Answer from the drawing. Dimensions are ordinates in mm from the lowest x, y and z of the part. A direction names the side the tool comes from. Coordinates: 2 decimals unless noted, no trailing zeros. Write each loop counter-clockwise with the first axis right and the second up, starting at its lowest first coordinate (ties: lowest second). Pieces come first, ordered by that corner, then holes. Notation, with made-up numbers: (25, -16.75) -> (56, -16.75) arc R9 ccw to (56, -5.75) -> close; hole circle Ø10 at (1.5, 55). An arc over 180 degrees is marked (long way). One line per item, written item: value. Start each with the question number.
1. Find section A-A, the plane z = 3.5. Write down the section's boundary in (x, y), and give its area (3 significant figures).
2. Consider line 1 along X through (y, z) = (2.65, 32.5); line 2 along Z through (x, y) = (16.25, 3.75); line 3 along Z through (x, y) = (6.75, 2.75). Determine where each line is inside the solid, lowest interval first.
3. For the marked faces 1, 2 and 3, determine the directions among +Z, -Z, +X, -X, +Y, -Y from which every point of the face is accessible in a straight line to the end or side of a thin tool.
4. Find section B-B, the plane x = 16. State how many separate pieces and enclosed holes the cut face has, and give its area (3 significant figures).
5. Given P1, Ø0.9, axis at x = 8, y = 5, coming from the -Z side; P2, Ø3, axis at x = 12, z = 4, coming from the +Y side; P3, Ø1, axis at x = 8, z = 21.5, coming from the -Y side; P4, Ø3, axis at x = 4, z = 32.5, coming from the +Y side, each flat-ended and moving along its own axis, determine where each tip first touches the part or whether it passes through.
6. Find section C-C, the plane y = 3.5. Write down the section's boundary in (x, z).
7. Find section D-D, the plane x = 13.5. Write down the section's boundary in (y, z).
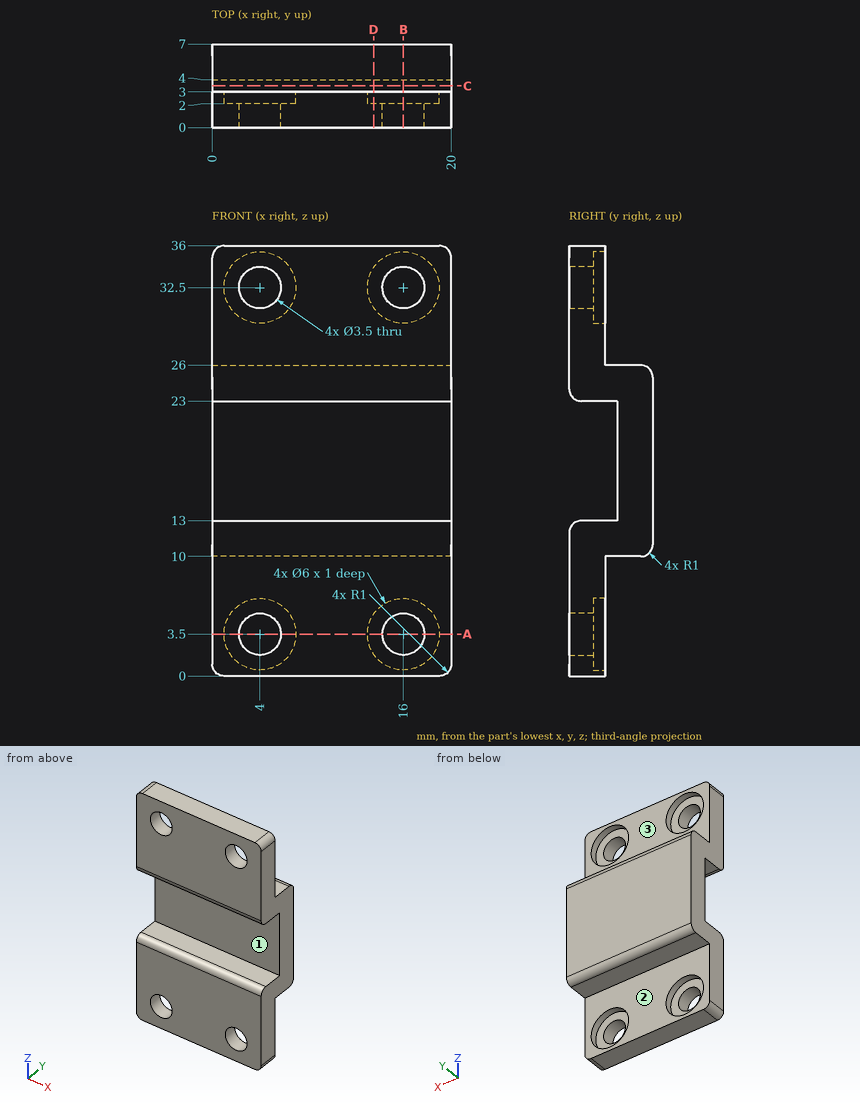
Answer block:
1. outline: (0, 0) -> (2.25, 0) -> (2.25, 2) -> (1, 2) -> (1, 3) -> (0, 3) -> close; (5.75, 0) -> (14.25, 0) -> (14.25, 2) -> (13, 2) -> (13, 3) -> (7, 3) -> (7, 2) -> (5.75, 2) -> close; (17.75, 0) -> (20, 0) -> (20, 3) -> (19, 3) -> (19, 2) -> (17.75, 2) -> close
1. area: 34.0 mm2
2. line 1: x = 0 to 1, 7 to 13, 19 to 20
2. line 2: z = 10 to 13, 23 to 26
2. line 3: z = 0 to 2.3, 4.7 to 13, 23 to 31.3, 33.7 to 36
3. face 1: +X, -X, -Y
3. face 2: -Z, +X, -X, +Y
3. face 3: +Z, +X, -X, +Y
4. separate pieces: 3
4. enclosed holes: 0
4. area: 105 mm2
5. P1: stops at z = 10
5. P2: stops at y = 3
5. P3: stops at y = 4
5. P4: passes through
6. outline: (0, 10) -> (20, 10) -> (20, 13) -> (0, 13) -> close; (0, 23) -> (20, 23) -> (20, 26) -> (0, 26) -> close
7. outline: (0, 0) -> (3, 0) -> (3, 1.84) -> (2, 1.84) -> (2, 5.16) -> (3, 5.16) -> (3, 10) -> (6, 10) arc R1 ccw to (7, 11) -> (7, 25) arc R1 ccw to (6, 26) -> (3, 26) -> (3, 30.84) -> (2, 30.84) -> (2, 34.16) -> (3, 34.16) -> (3, 36) -> (0, 36) -> (0, 24) arc R1 ccw to (1, 23) -> (4, 23) -> (4, 13) -> (1, 13) arc R1 ccw to (0, 12) -> close
